Model file for the job. Use its own axes, mm. Face numbers are marked on the shaded views. A direction names the side the tool comes from. Coordinates: 2 decimals unless noted, no trailing zeros. Write each loop counter-clockwise with the first axis right and the second up, starting at its lowest first coordinate (ties: lowest second). Pieces come first, ordered by that corner, then holes. Notation, with made-up numbers: M 84,88.25 L 114,88.25 A22 cw 114,124.25 Z; hole C -36,9.25 d8. An arc over 180 degrees is marked long. Use CSV: the item, a comma, the result in double quotes. Start each with the question number.
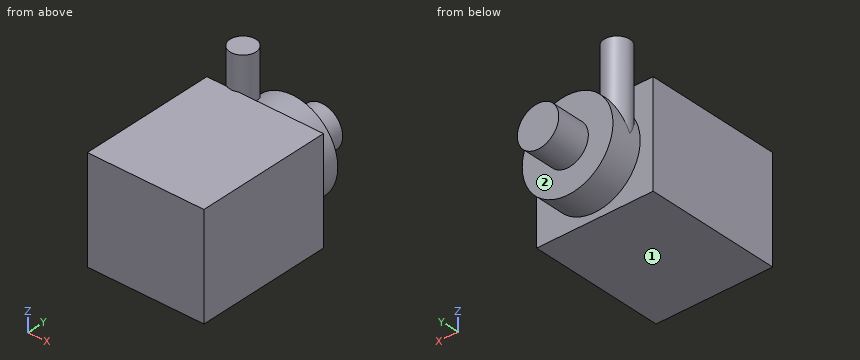
from build123d import *

# Parameters (mm, degrees)
F0_W     = 45
F0_H     = 40
F0_R     = 17.5
F0_R_2   = 8
F1_DEPTH = 52.6
F2_DEPTH = 12
F3_DEPTH = 25
F4_R     = 5
F5_DEPTH = 33


with BuildPart() as f1:
    # F0 (on Front) → F1 (new body)
    with BuildSketch(Plane.XZ):
        Rectangle(F0_W, F0_H)
        Circle(F0_R, mode=Mode.SUBTRACT)
        Circle(F0_R)
        Circle(F0_R_2, mode=Mode.SUBTRACT)
        Circle(F0_R_2)
    extrude(amount=F1_DEPTH)

    # F0 (on Front) → F2 (join)
    with BuildSketch(Plane.XZ):
        Circle(F0_R)
        Circle(F0_R_2, mode=Mode.SUBTRACT)
    extrude(amount=-F2_DEPTH)

    # F0 (on Front) → F3 (join)
    with BuildSketch(Plane.XZ):
        Circle(F0_R_2)
    extrude(amount=-F3_DEPTH)

    # F4 (on Top) → F5 (join)
    with BuildSketch(Plane.XY):
        with Locations((-12.5, 4.5)):
            Circle(F4_R)
    extrude(amount=F5_DEPTH)


solid = f1.part
1) Band-saw the part on A-A on x = 0. List the corners of the cut face in (y, z), then the cut area to 3 significant figures.
2) Band-saw the part on D-D on x = -12.5. List the corners of the cut face in (y, z), then the cut area to 3 significant figures.
3) Tool access for the marked faces 1 and 2: list every direction of +Z, -Z, +X, -X, +Y, -Y with a clear straight run to the whole face (end or side of a thin tool).
4) Band-saw the part on B-B on z = 12. List the corners of the cut face in (x, y), then the cut area to 3 significant figures.
5) Drop a flat-ended pin along its axis: P1, Ø1, axis at x = 0.5, y = 15.5, coming from the -Z side. Give the stop position or say it passes through.
6) Band-saw the part on C-C on y = -42. List the corners of the cut face in (x, z).
7) Wall check: L1, parallel to Z at x = -8.5, y = -6.5; L2, parallel to Y at x = 20, z = -14; L3, parallel to Y at x = -16, z = 9. Give the ranges that are in metal, low to high. Write a range as [from, to].
Findings below:
1,outline,"M -52.6,-20 L 0,-20 L 0,-17.5 L 12,-17.5 L 12,-8 L 25,-8 L 25,8 L 12,8 L 12,17.5 L 0,17.5 L 0,20 L -52.6,20 Z"
1,area,"2,730 mm2"
2,outline,"M -52.6,-20 L 0,-20 L 0,-12.25 L 12,-12.25 L 12,12.25 L 9.5,12.25 L 9.5,33 L -0.5,33 L -0.5,20 L -52.6,20 Z"
2,area,"2,600 mm2"
3,face 1,"-Z, +X, -X, +Y, -Y"
3,face 2,"+Y"
4,outline,"M -22.5,-52.6 L 22.5,-52.6 L 22.5,0 L 12.74,0 L 12.74,12 L -12.74,12 L -12.74,9.49 A5 ccw -14.68,0 L -22.5,0 Z"
4,area,"2,710 mm2"
5,P1,"stops at z = -8"
6,outline,"M -22.5,-20 L 22.5,-20 L 22.5,20 L -22.5,20 Z"
7,L1,"z = [-20, 20]"
7,L2,"y = [-52.6, 0]"
7,L3,"y = [-52.6, 0], [0.93, 8.07]"
